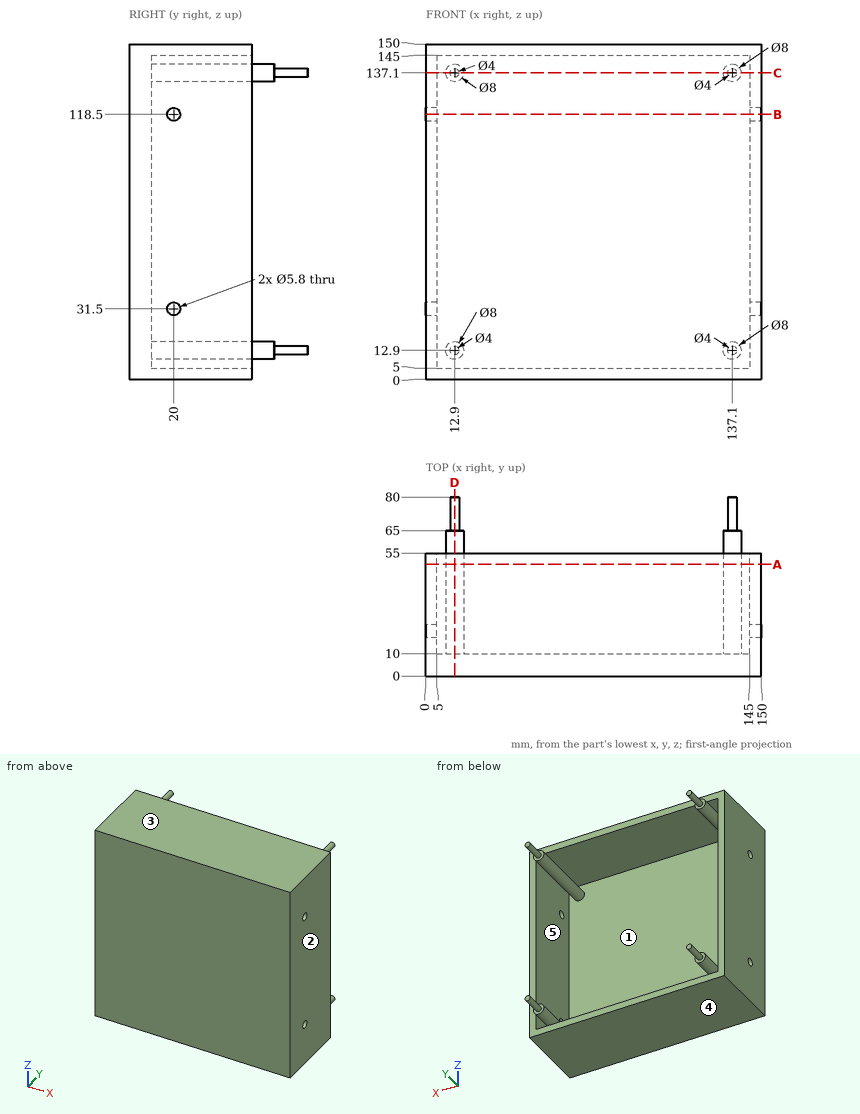
Design review of the part shown in the three views and the two pictorial views. Dimensions are in mm from the part's minimum x, y and z. A direction names the side the tool comes from. Round coordinates to 2 decimals unless told otherwise and drop trailing zeros. Write each loop counter-clockwise with the first axis right and the second up, starting at its lowest first coordinate (ties: lowest second). Pieces come first, ordered by that corner, then holes. Notation, with made-up numbers: (-29, -38.5) -> (-24, -38.5) arc R6 ccw to (-24, -33.5) -> close; hole circle Ø1 at (42.25, 23.25). An arc over 180 degrees is marked (long way). Write item = value, one per line. Start each with the question number.
1) Tool access review of the marked faces 1 and 2: name each direction out of +Z, -Z, +X, -X, +Y, -Y from which nothing blocks a thin tool from reaching the whole face with its end or side.
2) Take a section at B-B, the plane z = 118.5. State the section outline as (x, y) points.
3) Clearance check with flat-ended pins moving along their axes: pin 1 (1.5 mm diameter, centred on x = 64, z = 20, fed in from +Y); pin 2 (7.5 mm diameter, centred on y = 20, z = 118.5, fed in from +X); pin 3 (3.5 mm diameter, centred on y = 20, z = 118.5, fed in from -X). State where each tip first meets the part, or that it passes through.
4) Take a section at A-A, the plane y = 50. State the section outline as (x, z) points, plus the area to 3 significant figures.
5) Wall thickness on probe 1 along Z at (x, y) = (148.1, 20); probe 2 along X at (y, z) = (27, 39): over which ranges is each line inside the solid? List them lowest first. Write a range as from..to.
6) Take a section at D-D, the plane x = 12.9. State the section outline as (y, z) points, plus the area to 3 significant figures.
7) Take a section at C-C, the plane z = 137.1. State the section outline as (x, y) points.
8) Mouldability with a two-part tool opening along Z and no side actions: class the marked faces 3, 4 and 5 as +Z half, -Z half, draft (parallel to the pull), parting line (faces both ways), or undercut.
Results list:
q1.face_1 = +Y
q1.face_2 = +Z, -Z, +X, +Y, -Y
q2.outline = (0, 0) -> (150, 0) -> (150, 17.1) -> (145, 17.1) -> (145, 10) -> (5, 10) -> (5, 17.1) -> (0, 17.1) -> close; (0, 22.9) -> (5, 22.9) -> (5, 55) -> (0, 55) -> close; (145, 22.9) -> (150, 22.9) -> (150, 55) -> (145, 55) -> close
q3.pin_1 = 10
q3.pin_2 = 150
q3.pin_3 = through
q4.outline = (0, 0) -> (150, 0) -> (150, 150) -> (0, 150) -> close; circle Ø8 at (12.9, 12.9); circle Ø8 at (12.9, 137.1); circle Ø8 at (137.1, 12.9); circle Ø8 at (137.1, 137.1); hole (5, 5) -> (145, 5) -> (145, 145) -> (5, 145) -> close
q4.area = 3,100 mm²
q5.probe_1 = 0..28.6, 34.4..115.6, 121.4..150
q5.probe_2 = 0..5, 145..150
q6.outline = (0, 0) -> (55, 0) -> (55, 5) -> (10, 5) -> (10, 8.9) -> (65, 8.9) -> (65, 10.9) -> (80, 10.9) -> (80, 14.9) -> (65, 14.9) -> (65, 16.9) -> (10, 16.9) -> (10, 133.1) -> (65, 133.1) -> (65, 135.1) -> (80, 135.1) -> (80, 139.1) -> (65, 139.1) -> (65, 141.1) -> (10, 141.1) -> (10, 145) -> (55, 145) -> (55, 150) -> (0, 150) -> close
q6.area = 2,950 mm²
q7.outline = (0, 0) -> (150, 0) -> (150, 55) -> (145, 55) -> (145, 10) -> (141.1, 10) -> (141.1, 65) -> (139.1, 65) -> (139.1, 80) -> (135.1, 80) -> (135.1, 65) -> (133.1, 65) -> (133.1, 10) -> (16.9, 10) -> (16.9, 65) -> (14.9, 65) -> (14.9, 80) -> (10.9, 80) -> (10.9, 65) -> (8.9, 65) -> (8.9, 10) -> (5, 10) -> (5, 55) -> (0, 55) -> close
q8.face_3 = +Z half
q8.face_4 = -Z half
q8.face_5 = undercut
